Geometry: final body of the model. Coordinates: model frame, mm. A direction names the side the tool comes from. Round coordinates to 2 decimals unless told otherwise and drop trailing zeros. Write each loop counter-clockwise with the first axis right and the second up, starting at its lowest first coordinate (ties: lowest second). Pieces come first, ordered by that corner, then holes. Notation, with made-up numbers: (-27.5, -22.5) -> (-1.5, -22.5) arc R12 ccw to (-1.5, -13.5) -> close; hole circle Ø9 at (36, -16). An arc over 180 degrees is marked (long way). One line per item, written item: value. Start each with the question number.
from build123d import *

# Parameters (mm, degrees)
ESBO_O1_W                = 15
ESBO_O1_H                = 12
RESSALTO_EXTRUS_O1_DEPTH = 4
ESBO_O2_W                = 5.6
ESBO_O2_H                = 6
CORTE_EXTRUS_O1_DEPTH    = 11.404326023
ESBO_O3_W                = 1.2
ESBO_O3_H                = 10
CORTE_EXTRUS_O2_DEPTH    = 1
CHANFRO1_SIZE            = 0.5
FILETE1_R                = 2
FILETE2_R                = 2
FILETE3_R                = 2
FILETE4_R                = 2
ESBO_O4_W                = 1.2
ESBO_O4_H                = 10
CORTE_EXTRUS_O3_DEPTH    = 1
CHANFRO2_SIZE            = 0.5


with BuildPart() as part:
    # Esboço1 → Ressalto-extrusão1 (new body)
    with BuildSketch(Plane(origin=(0, 0, 0), x_dir=(1, 0, 0), z_dir=(0, 1, 0))):
        Rectangle(ESBO_O1_W, ESBO_O1_H)
    extrude(amount=RESSALTO_EXTRUS_O1_DEPTH)

    # Esboço2 → Corte-extrusão1 (cut, through all)
    with BuildSketch(Plane(origin=(0, 4, 0), x_dir=(1, 0, 0), z_dir=(0, 1, 0))):
        with Locations((0, 6)):
            Rectangle(ESBO_O2_W, ESBO_O2_H)
    extrude(amount=-CORTE_EXTRUS_O1_DEPTH, mode=Mode.SUBTRACT)

    # Esboço3 → Corte-extrusão2 (cut)
    with BuildSketch(Plane(origin=(0, 4, 0), x_dir=(1, 0, 0), z_dir=(0, 1, 0))):
        with Locations((0, -2)):
            Rectangle(ESBO_O3_W, ESBO_O3_H)
    extrude(amount=-CORTE_EXTRUS_O2_DEPTH, mode=Mode.SUBTRACT)

    # Chanfro1
    chanfro1_edges = [part.edges().sort_by_distance(p)[0] for p in [
        (0.6, 3, 1.5),
        (-0.6, 3, 1.5),
    ]]
    chamfer(chanfro1_edges, length=CHANFRO1_SIZE)

    # Filete1
    filete1_edges = [part.edges().sort_by_distance(p)[0] for p in [
        (7.5, 2, 6),
    ]]
    fillet(filete1_edges, radius=FILETE1_R)

    # Filete2
    filete2_edges = [part.edges().sort_by_distance(p)[0] for p in [
        (7.5, 2, -6),
    ]]
    fillet(filete2_edges, radius=FILETE2_R)

    # Filete3
    filete3_edges = [part.edges().sort_by_distance(p)[0] for p in [
        (-7.5, 2, 6),
    ]]
    fillet(filete3_edges, radius=FILETE3_R)

    # Filete4
    filete4_edges = [part.edges().sort_by_distance(p)[0] for p in [
        (-7.5, 2, -6),
    ]]
    fillet(filete4_edges, radius=FILETE4_R)

    # Esboço4 → Corte-extrusão3 (cut)
    with BuildSketch(Plane.XZ):
        with Locations((0, 2)):
            Rectangle(ESBO_O4_W, ESBO_O4_H)
    extrude(amount=-CORTE_EXTRUS_O3_DEPTH, mode=Mode.SUBTRACT)

    # Chanfro2
    chanfro2_edges = [part.edges().sort_by_distance(p)[0] for p in [
        (0.6, 1, 1.5),
        (-0.6, 1, 1.5),
    ]]
    chamfer(chanfro2_edges, length=CHANFRO2_SIZE)


solid = part.part
(1) Pull-direction query (X, two-part tool) for faces 3 (the face through (-4, 2, -6)), 4 (the face through (6.9, 2.03, 5.43)), 5 (the face through (0, 2, -3)); classes: pulls with the +X half, pulls with the -X half, needs draft (parallel to the pull), parting line crosses it, or undercut.
(2) Section query C-C (y = 1.55). Output: boundary loops of the cut face in (x, z), and give its area (3 significant figures).
(3) Line query: probe 1 along Z at (x, y) = (1.75, 1.65); probe 2 along X at (y, z) = (3.15, 2.25); probe 3 along X at (y, z) = (3.7, -5.5). Output: solid intervals per line, ascending.
(4) Set-up query: faces 1 (the face through (-4, 0, 0)), 2 (the face through (2.8, 2, -4)). Return all of +Z, -Z, +X, -X, +Y, -Y with unobstructed straight access to the full face (end or side cutting, diameter ignored); none if empty.
(5) Section query D-D (x = 1.5). Output: boundary loops of the cut face in (y, z), and give its area (3 significant figures).
(6) Section query B-B (z = 2). Output: boundary loops of the cut face in (x, y).
(7) Pin query (flat end, axial travel): pin 1 (1 mm diameter, centred on x = -2, y = 1.5, fed in from -Z). Return the tip coordinate at first contact, or that it passes through.
(8) Section query A-A (y = 0.75). Output: boundary loops of the cut face in (x, z).
Results list:
1. face 3: needs draft
1. face 4: pulls with the +X half
1. face 5: undercut
2. outline: (-7.5, -4) arc R2 ccw to (-5.5, -6) -> (-2.8, -6) -> (-2.8, -3) -> (2.8, -3) -> (2.8, -6) -> (5.5, -6) arc R2 ccw to (7.5, -4) -> (7.5, 4) arc R2 ccw to (5.5, 6) -> (-5.5, 6) arc R2 ccw to (-7.5, 4) -> close
2. area: 160 mm^2
3. probe 1: z = -3 to 6
3. probe 2: x = -7.5 to -0.25, 0.25 to 7.5
3. probe 3: x = -6.82 to -2.8, 2.8 to 6.82
4. face 1: +Z, -Z, +X, -X, -Y
4. face 2: -Z, +Y, -Y
5. outline: (0, -3) -> (4, -3) -> (4, 6) -> (0, 6) -> close
5. area: 36.0 mm^2
6. outline: (-7.5, 0) -> (-0.6, 0) -> (-0.6, 0.5) -> (-0.1, 1) -> (0.1, 1) -> (0.6, 0.5) -> (0.6, 0) -> (7.5, 0) -> (7.5, 4) -> (0.6, 4) -> (0.6, 3.5) -> (0.1, 3) -> (-0.1, 3) -> (-0.6, 3.5) -> (-0.6, 4) -> (-7.5, 4) -> close
7. pin 1: stops at z = -3
8. outline: (-7.5, -4) arc R2 ccw to (-5.5, -6) -> (-2.8, -6) -> (-2.8, -3) -> (-0.35, -3) -> (-0.35, 6) -> (-5.5, 6) arc R2 ccw to (-7.5, 4) -> close; (0.35, -3) -> (2.8, -3) -> (2.8, -6) -> (5.5, -6) arc R2 ccw to (7.5, -4) -> (7.5, 4) arc R2 ccw to (5.5, 6) -> (0.35, 6) -> close
